```python
from build123d import *

# Parameters (mm, degrees)
BOSS_EXTRUDE1_DEPTH       = 8.2
CUT_EXTRUDE1_DEPTH        = 2.2
SKETCH3_W                 = 6.75
SKETCH3_H                 = 8.2
BOSS_EXTRUDE2_DEPTH       = 4
F_1_5MM_DOWEL_HOLE1_D     = 1.5
F_1_5MM_DOWEL_HOLE1_DEPTH = 3
F_1_5MM_DOWEL_HOLE1_TIP   = 0.450645464
M2X0_4_TAPPED_HOLE1_D     = 1.6
M2X0_4_TAPPED_HOLE1_DEPTH = 4
M2X0_4_TAPPED_HOLE1_TIP   = 0.480688495


with BuildPart() as part:
    # Sketch1 → Boss-Extrude1 (new body)
    with BuildSketch(Plane.XY):
        Polygon((0, 0), (0, 4.787274917), (1.582547561, 6.315523332), (5.75, 2), (6.75, 2), (6.75, 0), align=None)
    extrude(amount=BOSS_EXTRUDE1_DEPTH)

    # Sketch2 → Cut-Extrude1 (cut)
    with BuildSketch(Plane(origin=(3.97472688, 3.838349131, 0), x_dir=(0, 0, -1), z_dir=(0.7193398, 0.69465837, 0))):
        with BuildLine():
            Line((-8.2, 3.443677383), (-2, 3.443677383))
            Line((-2, 3.443677383), (-2, -0.555606029))
            Line((-2, -0.555606029), (-1.75, -0.555606029))
            ThreePointArc((-1.75, -0.555606029), (-0.75, -1.555606029), (-1.75, -2.555606029))
            Line((-1.75, -2.555606029), (-8.2, -2.555606029))
            Line((-8.2, -2.555606029), (-8.2, 3.443677383))
        make_face()
    extrude(amount=-CUT_EXTRUDE1_DEPTH, mode=Mode.SUBTRACT)

    # Sketch3 → Boss-Extrude2 (add)
    with BuildSketch(Plane.XZ):
        with Locations((3.375, 4.1)):
            Rectangle(SKETCH3_W, SKETCH3_H)
    extrude(amount=BOSS_EXTRUDE2_DEPTH)

    # Ø1.5mm Dowel Hole1
    with Locations(Plane(origin=(0, -4, 0), x_dir=(-1, 0, 0), z_dir=(0, -1, 0))):
        with Locations((-2, -7.1), (-2, -1.1)):
            Hole(F_1_5MM_DOWEL_HOLE1_D / 2, depth=F_1_5MM_DOWEL_HOLE1_DEPTH)
            with Locations((0, 0, -(F_1_5MM_DOWEL_HOLE1_DEPTH + F_1_5MM_DOWEL_HOLE1_TIP / 2))):  # 118° drill point
                Cone(0, F_1_5MM_DOWEL_HOLE1_D / 2, F_1_5MM_DOWEL_HOLE1_TIP, mode=Mode.SUBTRACT)

    # M2x0.4 Tapped Hole1
    with Locations(Plane(origin=(0, -4, 0), x_dir=(-1, 0, 0), z_dir=(0, -1, 0))):
        with Locations((-2, -4.1)):
            Hole(M2X0_4_TAPPED_HOLE1_D / 2, depth=M2X0_4_TAPPED_HOLE1_DEPTH)
            with Locations((0, 0, -(M2X0_4_TAPPED_HOLE1_DEPTH + M2X0_4_TAPPED_HOLE1_TIP / 2))):  # 118° drill point
                Cone(0, M2X0_4_TAPPED_HOLE1_D / 2, M2X0_4_TAPPED_HOLE1_TIP, mode=Mode.SUBTRACT)


solid = part.part
```
The listing builds one solid part. Answer for the finished solid, in the listing's coordinates (mm). A direction names the side the tool comes from. Give positions to 0.01 mm unless a question says otherwise; leave off trailing zeros. Order: outer loops, then holes, each group sorted by start corner. A loop starts at its lowest first (then second) coordinate and runs counter-clockwise, first axis right, second up. Notation, with made-up numbers: (-31, 9) -> (14, 9) arc R26 ccw to (14, 32) -> close; hole circle Ø1 at (88.25, 42.25). An arc over 180 degrees is marked (long way). Answer as CSV lines item,"result". Start each with the question number.
Q1. A cutting plane is placed at C-C (z = 5.25). Determine the outline of the cut face in (x, y), then the cut area to 3 significant figures.
Q2. Determine the mould class of faces 1 (the flat face through (2.055, 2.66, 5.251)), 2 (the flat face through (3, -1, 8.2)), 3 (the flat face through (3.17, 4.67, 0.99)), 4 (the flat face through (0, 0, 4)) for opening direction X: pulls with the +X half, pulls with the -X half, needs draft (parallel to the pull), parting line crosses it, or undercut.
Q3. Find the intervals of material crossed by L1, parallel to Z at x = 2, y = -3.35; L2, parallel to X at y = -1.55, z = 4.1; L3, parallel to Y at x = 6, z = 4.5, in increasing order.
Q4. A cutting plane is placed at D-D (x = 6.25). Determine the outline of the cut face in (y, z).
Q5. A cutting plane is placed at B-B (y = -0.25). Determine the outline of the cut face in (x, z), then the cut area to 3 significant figures.
Q6. Which of the six approach directions +Z, -Z, +X, -X, +Y, -Y give full straight-line access (tool end or side, diameter ignored) to faces 5 (the cylindrical face through (2.346, -2.479, 7.765)), 6 (the flat face through (6, 2, 4)), 7 (the flat face through (3, -4, 4))?
Q7. Given pin 1 (0.5 mm diameter, centred on x = 6, z = 2, fed in from +Y); pin 2 (2.5 mm diameter, centred on x = 2, z = 4.1, fed in from +Y), each flat-ended and moving along its own axis, determine where each tip first touches the part or whether it passes through.
Q8. A cutting plane is placed at A-A (y = -2.5). Determine the outline of the cut face in (x, z).
Results found:
1,outline,"(0, -4) -> (6.75, -4) -> (6.75, 2) -> (5.75, 2) -> (4.17, 0.47) -> (0, 4.79) -> close"
1,area,"41.9 mm2"
2,face 1,"undercut"
2,face 2,"needs draft"
2,face 3,"pulls with the +X half"
2,face 4,"pulls with the -X half"
3,L1,"0 to 0.35, 1.85 to 3.3, 4.9 to 6.35, 7.85 to 8.2"
3,L2,"0 to 1.2, 2.8 to 6.75"
3,L3,"-4 to 2"
4,outline,"(-4, 0) -> (2, 0) -> (2, 8.2) -> (-4, 8.2) -> close"
5,outline,"(0, 0) -> (6.75, 0) -> (6.75, 8.2) -> (0, 8.2) -> close; hole circle Ø1.6 at (2, 4.1)"
5,area,"53.3 mm2"
6,face 5,"-Y"
6,face 6,"+Z, -Z, +X, +Y"
6,face 7,"+Z, -Z, +X, -X, -Y"
7,pin 1,"y = 2"
7,pin 2,"y = 4.01"
8,outline,"(0, 0) -> (6.75, 0) -> (6.75, 8.2) -> (0, 8.2) -> close; hole circle Ø1.6 at (2, 4.1); hole circle Ø1.5 at (2, 1.1); hole circle Ø1.5 at (2, 7.1)"
